```python
from build123d import *

# Parameters (mm, degrees)
CYLINDER_R      = 3.5
CYLINDER_DEPTH  = 3.82
SKETCH002_R     = 2
PAD001_DEPTH    = 50
POCKET001_DEPTH = 3


with BuildPart() as part:
    # Cylinder → Cylinder (new body)
    with BuildSketch(Plane.XY):
        Circle(CYLINDER_R)
    extrude(amount=CYLINDER_DEPTH)

    # Sketch002 → Pad001 (new body)
    with BuildSketch(Plane.XY.offset(3.82)):
        Circle(SKETCH002_R)
    extrude(amount=PAD001_DEPTH)

    # Sketch003 → Pocket001 (cut)
    with BuildSketch(Plane(origin=(0, 0, 0), x_dir=(1, 0, 0), z_dir=(0, 0, -1))):
        Polygon((1.732051, 1), (0, 2), (-1.732051, 1), (-1.732051, -1), (0, -2), (1.732051, -1), align=None)
    extrude(amount=-POCKET001_DEPTH, mode=Mode.SUBTRACT)


solid = part.part
```
Can you work these out from the model? Positions are in its coordinate system, mm. A direction names the side the tool comes from. Coordinates: 2 decimals unless noted, no trailing zeros. Loops run counter-clockwise (first coordinate to the right, second up) from the corner with the lowest first, then second, coordinate; pieces in that order, holes last.
1) I need wall thicknesses on probe 1 along Z at (x, y) = (0.25, -1.5); probe 2 along Z at (x, y) = (3, 0); probe 3 along Y at (x, z) = (-1, 13.5). Which ranges of each line are inside material? Lowest first, please.
2) Thinking about a two-plate mould opening in Y: for faces 4 (the flat face through (0.85, 1.51, 1.48)), 5 (the cylindrical face through (3.233, -1.341, 1.883)), 6 (the flat face through (0, 0, 53.82)), 7 (the flat face through (0, 0, 3)), which applies, pulls with the +Y half, pulls with the -Y half, needs draft (parallel to the pull), parting line crosses it, or undercut?
3) Imagine slicing it at C-C on x = 3. List the corners of the cut face in (y, z) for me.
4) Imagine slicing it at A-A on y = 0. List the corners of the cut face in (x, z) for me, plus the area to 3 significant figures.
5) For pin 1 (1.5 mm diameter, centred on x = 2.5, y = -2.5, fed in from +Z); pin 2 (0.6 mm diameter, centred on y = -0.5, z = 1.5, fed in from -X); pin 3 (1 mm diameter, centred on x = 0, y = 0, fed in from -Z), each with a flat end and sliding along its axis, tell me the tip position at first contact or that it passes through.
6) Imagine slicing it at B-B on z = 40. List the corners of the cut face in (x, y) for me.
7) Which directions (+Z, -Z, +X, -X, +Y, -Y) give clear straight access to the entire face, cutting with the end or side of a thin tool? Please do faces 1 (the flat face through (-0.85, -1.51, 1.48)), 2 (the cylindrical face through (0, -2, 28)), 3 (the flat face through (1, 2, 0)).
Completed:
1. probe 1: z = 3 to 53.82
1. probe 2: z = 0 to 3.82
1. probe 3: y = -1.73 to 1.73
2. face 4: undercut
2. face 5: parting line crosses it
2. face 6: needs draft
2. face 7: undercut
3. outline: (-1.8, 0) - (1.8, 0) - (1.8, 3.82) - (-1.8, 3.82) - close
4. outline: (-3.5, 0) - (-1.73, 0) - (-1.73, 3) - (1.73, 3) - (1.73, 0) - (3.5, 0) - (3.5, 3.82) - (2, 3.82) - (2, 53.82) - (-2, 53.82) - (-2, 3.82) - (-3.5, 3.82) - close
4. area: 216 mm2
5. pin 1: stops at z = 3.82
5. pin 2: stops at x = -3.49
5. pin 3: stops at z = 3
6. outline: circle Ø4 at (0, 0)
7. face 1: -Z
7. face 2: +Z
7. face 3: -Z, +X, -X, +Y, -Y
